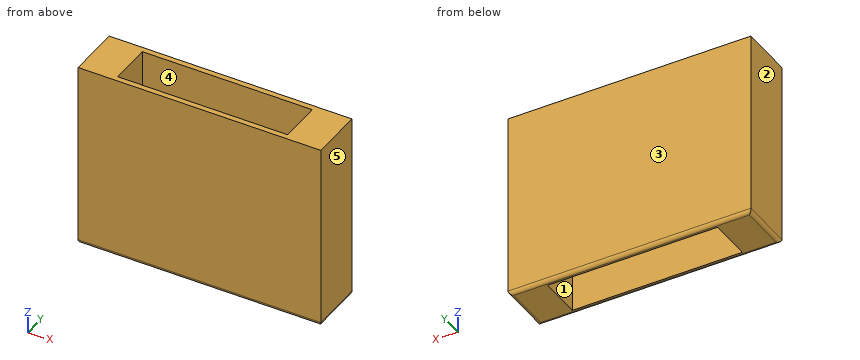
```python
from build123d import *

# Parameters (mm, degrees)
F0_W     = 50.8
F0_H     = 39.37
F1_DEPTH = 5.588
F2_W     = 35.56
F2_H     = 8.89
F3_DEPTH = 39.37
F4_R     = 0.762


with BuildPart() as f1:
    # F0 (on Front) → F1 (new body, symmetric)
    with BuildSketch(Plane.XZ):
        Rectangle(F0_W, F0_H)
    extrude(amount=F1_DEPTH, both=True)

    # F2 (on face) → F3 (cut)
    with BuildSketch(Plane.XY.offset(19.685)):
        Rectangle(F2_W, F2_H)
    extrude(amount=-F3_DEPTH, mode=Mode.SUBTRACT)

    # F4
    f4_edges = [f1.edges().sort_by_distance(p)[0] for p in [
        (25.4, 0, -19.685),
        (0, -5.588, -19.685),
        (0, 5.588, -19.685),
        (-25.4, 0, -19.685),
    ]]
    fillet(f4_edges, radius=F4_R)


solid = f1.part
```
For this review, take the finished solid that the model builds, in its own axes (mm). Face numbers are marked on the shaded views. A direction names the side the tool comes from. Give positions to 0.01 mm unless a question says otherwise; leave off trailing zeros. Write each loop counter-clockwise with the first axis right and the second up, starting at its lowest first coordinate (ties: lowest second). Pieces come first, ordered by that corner, then holes. Notation, with made-up numbers: M 2.5,85 L 15.5,85 A15 cw 15.5,95 Z; hole C 82,-15 d7. An arc over 180 degrees is marked long. Answer as CSV lines item,"result".
1. Wall thickness on line 1 (X direction, y = -3, z = 14.5); line 2 (Y direction, x = 15, z = 18) (3 decimals); line 3 (Z direction, x = -23, y = 5.25) (3 decimals): over which ranges is each line inside the solid? List them lowest first.
Findings:
line 1,"x = -25.4 to -17.78, 17.78 to 25.4"
line 2,"y = -5.588 to -4.445, 4.445 to 5.588"
line 3,"z = -19.556 to 19.685"
2. Draft analysis for pull direction X (two halves, no side actions). For the marked faces 3, 4 and 5, state which applies: +X half, -X half, draft (parallel to the pull), parting line (faces both ways), or undercut.
Findings:
face 3,"draft"
face 4,"undercut"
face 5,"+X half"
3. Consider section C-C, the plane z = -6. Write out the cut boundary in (x, y) (3 decimals), then the cut area to 3 significant figures.
Findings:
outline,"M -25.4,-5.588 L 25.4,-5.588 L 25.4,5.588 L -25.4,5.588 Z; hole M -17.78,-4.445 L 17.78,-4.445 L 17.78,4.445 L -17.78,4.445 Z"
area,"252 mm2"
4. Consider section B-B, the plane x = -13. Write out the cut boundary in (y, z) (3 decimals).
Findings:
outline,"M -5.588,-18.923 A0.762 ccw -4.826,-19.685 L -4.445,-19.685 L -4.445,19.685 L -5.588,19.685 Z; M 4.445,-19.685 L 4.826,-19.685 A0.762 ccw 5.588,-18.923 L 5.588,19.685 L 4.445,19.685 Z"
5. For the marked faces 1 and 2, list the 3-axis set-ups (+Z, -Z, +X, -X, +Y, -Y) from which the entire face can be reached by the end or side of a thin tool; tool diameter is ignored.
Findings:
face 1,"+Z, -Z"
face 2,"+Z, -Z, -X, +Y, -Y"
6. Consider section A-A, the plane y = 2.25. Write out the cut boundary in (x, z) (3 decimals), then the cut area to 3 significant figures.
Findings:
outline,"M -25.4,-18.923 A0.762 ccw -24.638,-19.685 L -17.78,-19.685 L -17.78,19.685 L -25.4,19.685 Z; M 17.78,-19.685 L 24.638,-19.685 A0.762 ccw 25.4,-18.923 L 25.4,19.685 L 17.78,19.685 Z"
area,"600 mm2"
